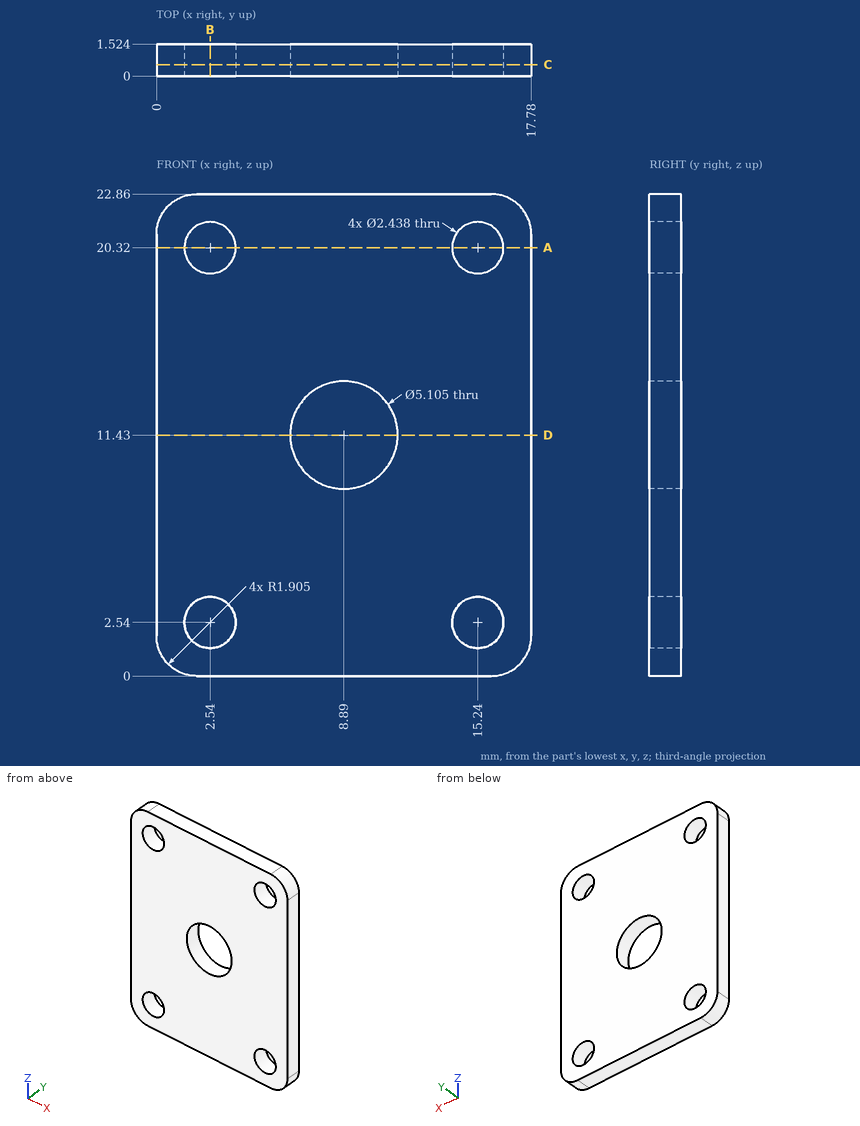
Could you check a few things on this drawing? It's one solid part, dimensions in mm from its lowest x, y, z. Give positions to 0.01 mm unless a question says otherwise; leave off trailing zeros. Write each loop counter-clockwise with the first axis right and the second up, starting at its lowest first coordinate (ties: lowest second). Pieces come first, ordered by that corner, then holes. Notation, with made-up numbers: (3, 60.25) -> (50, 60.25) arc R25 ccw to (50, 78.25) -> close; hole circle Ø9 at (-4.5, 24.25). An arc over 180 degrees is marked (long way). Answer as CSV lines item,"result". Start each with the question number.
(1) If we section it at D-D, the plane z = 11.43: Write out the boundary of the cut face in (x, y), and give its area (3 significant figures).
(2) I'm going to push a flat-ended pin straight in: pin 1 Ø4.5 at (x, z) = (8.89, 11.43) entering from -Y (3 decimals). Where does the tip first touch, or does it pass through?
(3) If we section it at A-A, the plane z = 20.32: Write out the boundary of the cut face in (x, y).
(4) If we section it at C-C, the plane y = 0.55: Write out the boundary of the cut face in (x, z) (1 decimal), and give its area (3 significant figures).
(5) Please list where these lines run through material, in increasing order: line 1 (X direction, y = 0.6, z = 20.32); line 2 (X direction, y = 1.25, z = 11.25); line 3 (Z direction, x = 8.89, y = 0.9).
(6) If we section it at B-B, the plane x = 2.54: Write out the boundary of the cut face in (y, z), and give its area (3 significant figures).
Answer list:
1,outline,"(0, 0) -> (6.34, 0) -> (6.34, 1.52) -> (0, 1.52) -> close; (11.44, 0) -> (17.78, 0) -> (17.78, 1.52) -> (11.44, 1.52) -> close"
1,area,"19.3 mm^2"
2,pin 1,"through"
3,outline,"(0, 0) -> (1.32, 0) -> (1.32, 1.52) -> (0, 1.52) -> close; (3.76, 0) -> (14.02, 0) -> (14.02, 1.52) -> (3.76, 1.52) -> close; (16.46, 0) -> (17.78, 0) -> (17.78, 1.52) -> (16.46, 1.52) -> close"
4,outline,"(0, 1.9) arc R1.9 ccw to (1.9, 0) -> (15.9, 0) arc R1.9 ccw to (17.8, 1.9) -> (17.8, 21) arc R1.9 ccw to (15.9, 22.9) -> (1.9, 22.9) arc R1.9 ccw to (0, 21) -> close; hole circle Ø2.4 at (2.5, 2.5); hole circle Ø2.4 at (2.5, 20.3); hole circle Ø5.1 at (8.9, 11.4); hole circle Ø2.4 at (15.2, 2.5); hole circle Ø2.4 at (15.2, 20.3)"
4,area,"364 mm^2"
5,line 1,"0 to 1.32, 3.76 to 14.02, 16.46 to 17.78"
5,line 2,"0 to 6.34, 11.44 to 17.78"
5,line 3,"0 to 8.88, 13.98 to 22.86"
6,outline,"(0, 0) -> (1.52, 0) -> (1.52, 1.32) -> (0, 1.32) -> close; (0, 3.76) -> (1.52, 3.76) -> (1.52, 19.1) -> (0, 19.1) -> close; (0, 21.54) -> (1.52, 21.54) -> (1.52, 22.86) -> (0, 22.86) -> close"
6,area,"27.4 mm^2"
